The listing builds one solid part. Answer for the finished solid, in the listing's coordinates (mm). Face numbers are marked on the shaded views. A direction names the side the tool comes from. Give positions to 0.01 mm unless a question says otherwise; leave off trailing zeros. Loops run counter-clockwise (first coordinate to the right, second up) from the corner with the lowest first, then second, coordinate; pieces in that order, holes last. Notation, with made-up numbers: M -14,-3 L 17,-3 A22 cw 17,11 Z; hole C 17,-4.75 d7. An arc over 180 degrees is marked long. One line per item, written item: value. Start each with the question number.
Q1. For the marked faces 4, 5 and 6, determine the directions among +Z, -Z, +X, -X, +Y, -Y from which every point of the face is accessible in a straight line to the end or side of a thin tool.
Q2. A cutting plane is placed at A-A, the plane x = 0. Determine the outline of the cut face in (y, z) (3 decimals).
Q3. Flat-ended cylindrical pins translate along their axes: pin 1 (1.6 mm diameter, centred on x = 1, y = 115, fed in from -Z); pin 2 (3 mm diameter, centred on x = 0, z = 4.5, fed in from -Y); pin 3 (1 mm diameter, centred on y = 116.5, z = 1, fed in from -X) (3 decimals). Find the tip coordinate at first contact, or state that the pin passes through.
Q4. A cutting plane is placed at C-C, the plane z = -4.5. Determine the outline of the cut face in (x, y) (3 decimals), and give its area (3 significant figures).
Q5. A cutting plane is placed at D-D, the plane z = -0.75. Determine the outline of the cut face in (x, y) (3 decimals), and give its area (3 significant figures).
Q6. The mould has two halves that part along X. Classify the marked faces 1, 2 and 3: +X half, -X half, draft (parallel to the pull), parting line (faces both ways), or undercut.
Q7. Consider L1, parallel to Z at x = -0.25, y = 114.9; L2, parallel to X at y = 114.85, z = 4.5 (3 decimals); L3, parallel to X at y = 114.9, z = 0.5 (3 decimals). Determine where each line is inside the solid, lowest interval first.
Q8. A cutting plane is placed at B-B, the plane y = 114.95. Determine the outline of the cut face in (x, z) (3 decimals).
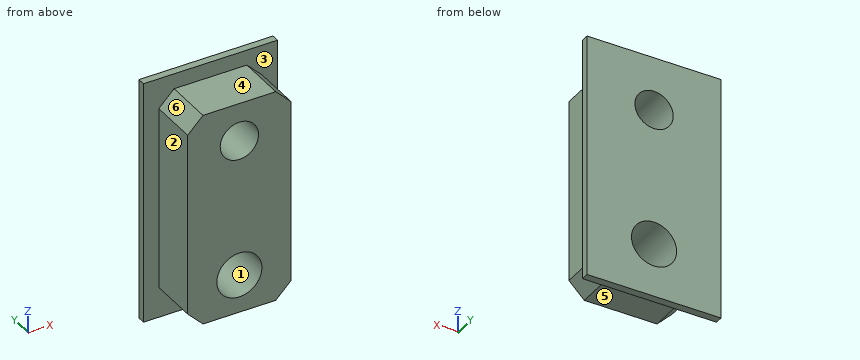
from build123d import *

# Parameters (mm, degrees)
SKETCH1_W             = 6.75
SKETCH1_H             = 3.175
EXTRUDE1_DEPTH        = 7
SKETCH6_W             = 8.75
SKETCH6_H             = 16
EXTRUDE2_DEPTH        = 0.5
F_4_CLEARANCE_HOLE1_D = 2.9464
SKETCH3_R             = 1.25
CUT_EXTRUDE1_DEPTH    = 4.675
CHAMFER1_SIZE         = 1


with BuildPart() as part:
    # Sketch1 → Extrude1 (new body, symmetric)
    with BuildSketch(Plane.XY):
        with Locations((0, 115.5875)):
            Rectangle(SKETCH1_W, SKETCH1_H)
    extrude(amount=EXTRUDE1_DEPTH, both=True)

    # Sketch6 → Extrude2 (add)
    with BuildSketch(Plane(origin=(0, 117.175, 0), x_dir=(1, 0, 0), z_dir=(0, 1, 0))):
        Rectangle(SKETCH6_W, SKETCH6_H)
    extrude(amount=EXTRUDE2_DEPTH)

    # 4 Clearance Hole1 (through all)
    with Locations(Plane(origin=(-0.355703292, 117.675, 3.885176073), x_dir=(-1, 0, 0), z_dir=(0, 1, 0))):
        with Locations((-0.355703292, -8.385176073)):
            Hole(F_4_CLEARANCE_HOLE1_D / 2)

    # Sketch3 → Cut-Extrude1 (cut, through all)
    with BuildSketch(Plane(origin=(0, 117.675, 0), x_dir=(1, 0, 0), z_dir=(0, 1, 0))):
        with Locations(Location((0, -4.5, 0), (0, 0, 270))):  # turned: the seam where the file's is
            Circle(SKETCH3_R)
    extrude(amount=-CUT_EXTRUDE1_DEPTH, mode=Mode.SUBTRACT)

    # Chamfer1
    chamfer1_edges = [part.edges().sort_by_distance(p)[0] for p in [
        (-3.375, 115.5875, 7),
        (-3.375, 115.5875, -7),
        (3.375, 115.5875, -7),
        (3.375, 115.5875, 7),
    ]]
    chamfer(chamfer1_edges, length=CHAMFER1_SIZE)


solid = part.part
Answer block:
1. face 4: +Z, +X, -X, -Y
1. face 5: -Z, +X, -X, -Y
1. face 6: +Z, -X, -Y
2. outline: M 114,-7 L 117.175,-7 L 117.175,-8 L 117.675,-8 L 117.675,-5.973 L 114,-5.973 Z; M 114,-3.027 L 117.675,-3.027 L 117.675,3.25 L 114,3.25 Z; M 114,5.75 L 117.675,5.75 L 117.675,8 L 117.175,8 L 117.175,7 L 114,7 Z
3. pin 1: z = -7
3. pin 2: y = 114
3. pin 3: x = -3.375
4. outline: M -4.375,117.175 L -3.375,117.175 L -3.375,114 L -1.473,114 L -1.473,117.675 L -4.375,117.675 Z; M 1.473,114 L 3.375,114 L 3.375,117.175 L 4.375,117.175 L 4.375,117.675 L 1.473,117.675 Z
4. area: 15.0 mm^2
5. outline: M -4.375,117.175 L -3.375,117.175 L -3.375,114 L 3.375,114 L 3.375,117.175 L 4.375,117.175 L 4.375,117.675 L -4.375,117.675 Z
5. area: 25.8 mm^2
6. face 1: undercut
6. face 2: -X half
6. face 3: draft
7. L1: -7 to -5.95, -3.05 to 3.28, 5.72 to 7
7. L2: -3.375 to -1.25, 1.25 to 3.375
7. L3: -3.375 to 3.375
8. outline: M -3.375,-6 L -2.375,-7 L 2.375,-7 L 3.375,-6 L 3.375,6 L 2.375,7 L -2.375,7 L -3.375,6 Z; hole C 0,-4.5 d2.946; hole C 0,4.5 d2.5
